Work out the finished part from the listing and answer in its coordinate system (mm). A direction names the side the tool comes from. Round coordinates to 2 decimals unless told otherwise and drop trailing zeros. Loops run counter-clockwise (first coordinate to the right, second up) from the corner with the lowest first, then second, coordinate; pieces in that order, holes last. Notation, with made-up numbers: (10.5, 31) -> (51.5, 31) arc R32 cw to (51.5, 65) -> close; hole circle Ø7 at (70.5, 0.25). An arc over 180 degrees is marked (long way). Use CSV: the item, a comma, the result in double quotes. Start each with the question number.
Autodesk Inventor part; units mm, degrees
ref_plane "YZ Plane" through (0, 0, 0) normal (1, 0, 0) x (0, 1, 0)
ref_plane "XZ Plane" through (0, 0, 0) normal (0, 1, 0) x (-1, 0, 0)
ref_plane "XY Plane" through (0, 0, 0) normal (0, 0, 1) x (1, 0, 0)
sketch "スケッチ1" plane through (0, 0, 0) normal (0, 0, 1) x (1, 0, 0)
  line L0 (-12.5, 25) -> (12.5, 25)
  line L1 (12.5, 25) -> (12.5, -25)
  line L2 (12.5, -25) -> (-12.5, -25)
  line L3 (-12.5, -25) -> (-12.5, 25)
  line L4 (-10.5, 23) -> (10.5, 23)
  line L5 (10.5, 23) -> (10.5, -23)
  line L6 (10.5, -23) -> (-10.5, -23)
  line L7 (-10.5, -23) -> (-10.5, 23)
  point P0 (0, 0)
  dimension "d0" = 25
  dimension "d1" = 50
  dimension "d2" = 46
  dimension "d3" = 21
  dimension "d4" = 25
  dimension "d5" = 23
  dimension "d6" = 10.5
  dimension "d7" = 12.5
extrude "押し出し1" add sketch "スケッチ1" along normal blind 50
sketch "スケッチ2" plane through (-12.5, 25, 0) normal (0, 1, 0) x (1, 0, 0)
  line L0 (0, 0) -> (25, 0)
  line L1 (0, 0) -> (0, -50)
  arc A0 (6, -33.5) -> (19, -33.5) centre (12.5, -33.5) ccw
  line L2 (6, -33.5) -> (6, 0)
  line L3 (19, -33.5) -> (19, 0)
  point P0 (12.5, 0)
  dimension "d10" = 13
  dimension "d11" = 33.5
  dimension "d12" = 12.5
extrude "押し出し2" cut sketch "スケッチ2" against normal blind 2
sketch "スケッチ3" plane through (-12.5, 25, 50) normal (0, 1, 0) x (1, 0, 0)
  arc A0 (6, 16.5) -> (19, 16.5) centre (12.5, 16.5) ccw
  circle A1 centre (4.5, 10) radius 1
  circle A2 centre (4.5, 46) radius 1
  circle A3 centre (20.5, 46) radius 1
  circle A4 centre (20.5, 10) radius 1
  point P0 (12.5, 50)
  dimension "d15" = 6.5
  dimension "d16" = 6.5
  dimension "d17" = 2
  dimension "d18" = 8
  dimension "d19" = 8
  dimension "d20" = 8
  dimension "d21" = 8
  dimension "d22" = 29.5
  dimension "d23" = 29.5
hole "穴1" at (-8, 25, 4) at (8, 25, 4) at (8, 25, 40) at (-8, 25, 40) direction (0, -1, 0) diameter 2 depth 2 tip angle 118 counterbore diameter 4 counterbore depth 0.5
sketch "スケッチ4" plane through (-12.5, -25, 0) normal (0, -1, 0) x (1, 0, 0)
  line L0 (25, 0) -> (0, 0)
  line L1 (25, 0) -> (25, 50)
  circle A0 centre (12.5, 10.5) radius 2
  point P0 (12.5, 0)
  dimension "d31" = 4
  dimension "d32" = 12.5
  dimension "d33" = 10.5
hole "穴2" at (0, -25, 10.5) direction (0, 1, 0) diameter 4 end through all
sketch "スケッチ5" plane through (-12.5, 25, 50) normal (0, 1, 0) x (1, 0, 0)
  line L0 (0, 0) -> (25, 0)
  arc A0 (6, 16.5) -> (19, 16.5) centre (12.5, 16.5) ccw
  circle A1 centre (20.5, 4) radius 1.5
  circle A2 centre (4.5, 4) radius 1.5
  point P0 (12.5, 50)
  dimension "d43" = 4
  dimension "d44" = 4
  dimension "d46" = 8
  dimension "d47" = 8
  dimension "d57" = 3
hole "穴4" at (-8, 25, 46) at (8, 25, 46) direction (0, -1, 0) diameter 3 end through all
thread "ねじ1"
thread "ねじ2"
thread "ねじ3"
thread "ねじ4"
sketch "スケッチ7" plane through (-12.5, -25, 0) normal (0, -1, 0) x (1, 0, 0)
  line L0 (25, 50) -> (0, 50)
  line L1 (0, 0) -> (0, 50)
  circle A0 centre (12.5, 30) radius 4
  point P0 (12.5, 0)
  dimension "d78" = 8
  dimension "d80" = 20
  dimension "d81" = 12.5
hole "穴5" at (0, -25, 30) direction (0, 1, 0) diameter 8 end through all
properties part number "08" material "アルミニウム 6061"
Q1. For a pull along X with two mould halves and no side action, classify faces 1 (the flat face through (-11, 2, 50)), 2 (the flat face through (12.5, 0, 25)), 3 (the cylindrical face through (-8.07, 23.99, 44.5)) as pulls with the +X half, pulls with the -X half, needs draft (parallel to the pull), parting line crosses it, or undercut.
Q2. Which of the six approach directions +Z, -Z, +X, -X, +Y, -Y give full straight-line access (tool end or side, diameter ignored) to faces 4 (the cylindrical face through (10, 24.75, 3.93)), 5 (the flat face through (-6.5, 24, 17)), 6 (the flat face through (-10.5, 0, 25)), 7 (the cylindrical face through (8.9, 24, 44.8))?
Q3. Section C-C, the plane y = 6 is taken. Write down the section's boundary in (x, z).
Q4. Each of these flat-tipped pins is pushed along its axis until it touches: pin 1 (2.5 mm diameter, centred on x = -8, z = 46, fed in from +Y); pin 2 (1 mm diameter, centred on x = 8.5, z = 3, fed in from +Y). Where does it stop, or does it pass through?
Q5. Section B-B, the plane x = -8 is taken. Give the number of separate pieces and of enclosed holes in the cut face, and give its area (3 significant figures).
Q6. Section A-A, the plane z = 10.5 is taken. Write down the section's boundary in (x, y).
Q7. Straight lines are drawn through the part: line 1 (X direction, y = 24, z = 4); line 2 (Z direction, x = 8, y = 23.95); line 3 (Z direction, x = -8, y = 24.85). For each, find the intervals that lie inside material, in ascending order. Write a range as from..to.
Q8. Section D-D, the plane z = 4 is taken. Write down the section's boundary in (x, y).
Report:
1,face 1,"needs draft"
1,face 2,"pulls with the +X half"
1,face 3,"undercut"
2,face 4,"+Y"
2,face 5,"-Z, +Y"
2,face 6,"+Z, -Z"
2,face 7,"+Y, -Y"
3,outline,"(-12.5, 0) -> (-10.5, 0) -> (-10.5, 50) -> (-12.5, 50) -> close; (10.5, 0) -> (12.5, 0) -> (12.5, 50) -> (10.5, 50) -> close"
4,pin 1,"passes through"
4,pin 2,"stops at y = 24.5"
5,separate pieces,"6"
5,enclosed holes,"0"
5,area,"178 mm²"
6,outline,"(-12.5, -25) -> (-2, -25) -> (-2, -23) -> (-10.5, -23) -> (-10.5, 23) -> (-6.5, 23) -> (-6.5, 25) -> (-12.5, 25) -> close; (2, -25) -> (12.5, -25) -> (12.5, 25) -> (6.5, 25) -> (6.5, 23) -> (10.5, 23) -> (10.5, -23) -> (2, -23) -> close"
7,line 1,"x = -12.5..-9, -7..-6.5, 6.5..7, 9..12.5"
7,line 2,"z = 0..3, 5..39, 41..44.5, 47.5..50"
7,line 3,"z = 0..2, 6..38, 42..44.5, 47.5..50"
8,outline,"(-12.5, -25) -> (12.5, -25) -> (12.5, 25) -> (10, 25) -> (10, 24.5) -> (9, 24.5) -> (9, 23) -> (10.5, 23) -> (10.5, -23) -> (-10.5, -23) -> (-10.5, 23) -> (-9, 23) -> (-9, 24.5) -> (-10, 24.5) -> (-10, 25) -> (-12.5, 25) -> close; (-7, 23) -> (-6.5, 23) -> (-6.5, 24.5) -> (-7, 24.5) -> close; (6.5, 23) -> (7, 23) -> (7, 24.5) -> (6.5, 24.5) -> close"
